Part print with two shaded views. Sizes in mm from the minimum x, y, z corner. A direction names the side the tool comes from. Give positions to 0.01 mm unless a question says otherwise; leave off trailing zeros. Order: outer loops, then holes, each group sorted by start corner. A loop starts at its lowest first (then second) coordinate and runs counter-clockwise, first axis right, second up. Notation, with made-up numbers: M 34,-18 L 47,-18 A9 ccw 47,-13 Z; hole C 77.25,5 d10. An arc over 180 degrees is marked long. Return JSON: item names as keys, results as strings.
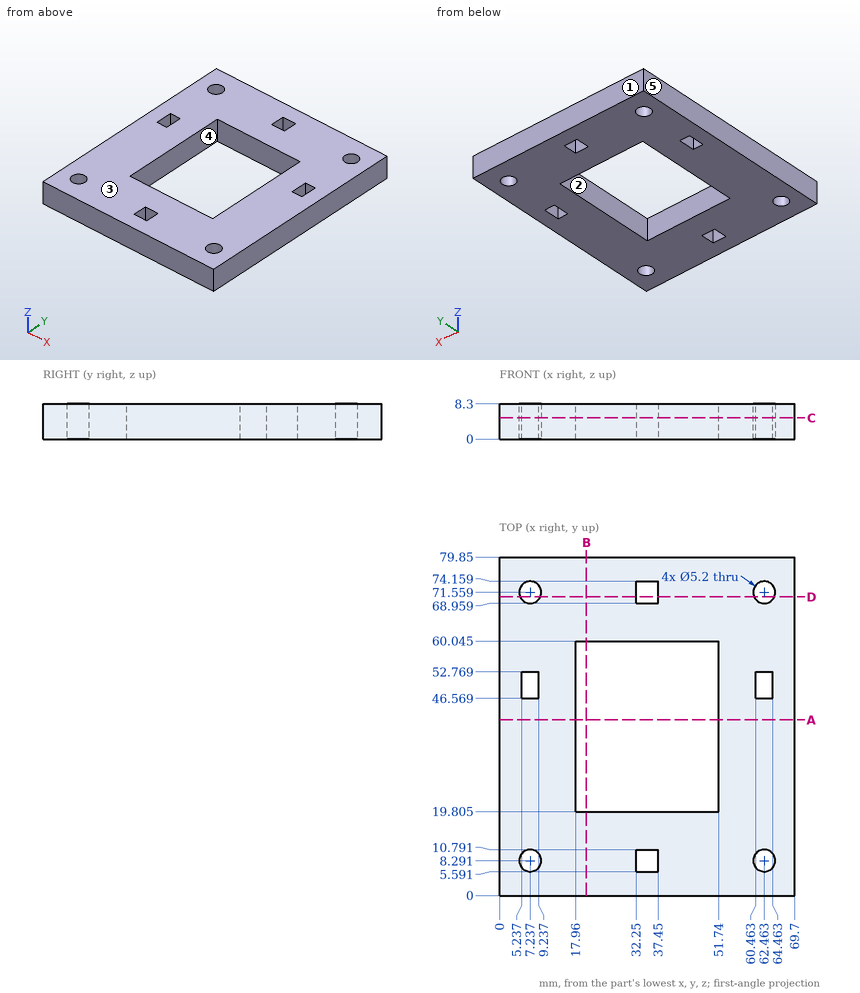
Q1. 3-axis set-ups, long thin cutter, end or side, ignore diameter. For the marked faces 4 and 5: which of +Z, -Z, +X, -X, +Y, -Y reach the whole face in a straight line?
Established:
{"face 4": "+Z, -Z", "face 5": "+Z, -Z, -X, +Y, -Y"}
Q2. Band-saw the part on C-C (z = 5). Give the number of separate pieces and of enclosed holes in the cut face, then the cut area to 3 significant figures.
Established:
{"separate pieces": "1", "enclosed holes": "9", "area": "4,020 mm²"}
Q3. Band-saw the part on A-A (y = 41.5). Give the cut face in (x, z), then the cut area to 3 significant figures.
Established:
{"outline": "M 0,0 L 17.96,0 L 17.96,8.3 L 0,8.3 Z; M 51.74,0 L 69.7,0 L 69.7,8.3 L 51.74,8.3 Z", "area": "298 mm²"}
Q4. Pin check, flat tip, straight feed: pin 1 (4.5 mm diameter, centred on x = 7.24, y = 71.56, fed in from -Z). Stop position of the tip, or through.
Established:
{"pin 1": "passes through"}
Q5. Two-plate mould, pull along Y, no slides. Class the marked faces 1, 2 and 3: +Y half, -Y half, draft (parallel to the pull), parting line (faces both ways), or undercut.
Established:
{"face 1": "+Y half", "face 2": "undercut", "face 3": "draft"}
Q6. Band-saw the part on B-B (x = 20.5). Give the cut face in (y, z) (3 decimals), then the cut area to 3 significant figures.
Established:
{"outline": "M 0,0 L 19.805,0 L 19.805,8.3 L 0,8.3 Z; M 60.045,0 L 79.85,0 L 79.85,8.3 L 60.045,8.3 Z", "area": "329 mm²"}
Q7. Probe line 1 along X through (y, z) = (50, 3.5); line 2 along X through (y, z) = (32.5, 1.25); line 3 along Y through (x, z) = (40, 2) (3 decimals). List the from-to ranges inside material, lowest first.
Established:
{"line 1": "x = 0 to 5.24, 9.24 to 17.96, 51.74 to 60.46, 64.46 to 69.7", "line 2": "x = 0 to 17.96, 51.74 to 69.7", "line 3": "y = 0 to 19.805, 60.045 to 79.85"}
Q8. Band-saw the part on D-D (y = 70.5). Give the cut face in (x, z).
Established:
{"outline": "M 0,0 L 4.86,0 L 4.86,8.3 L 0,8.3 Z; M 9.61,0 L 32.25,0 L 32.25,8.3 L 9.61,8.3 Z; M 37.45,0 L 60.09,0 L 60.09,8.3 L 37.45,8.3 Z; M 64.84,0 L 69.7,0 L 69.7,8.3 L 64.84,8.3 Z"}
